Work out the finished part from the listing and answer in its coordinate system (mm). A direction names the side the tool comes from. Round coordinates to 2 decimals unless told otherwise and drop trailing zeros. Write each loop counter-clockwise with the first axis right and the second up, starting at its lowest first coordinate (ties: lowest second). Pieces come first, ordered by that corner, then holes. Notation, with made-up numbers: (11, -15.75) - (49, -15.75) arc R11 ccw to (49, -1.75) - close; hole circle Ø6 at (6, 32). An arc over 180 degrees is marked (long way). Write item = value, one per line. Start each with the question number.
from build123d import *

# Parameters (mm, degrees)
SKETCH_1_R                   = 21.5
EXTRUDE_1_DEPTH              = 12
EXTRUDE_START                = -13.5
EXTRUDE_2_DEPTH              = 13.5
FILLET_1_R                   = 10
SKETCH_4_R                   = 20
CUT_EXTRUDE_1_DEPTH          = 6
SKETCH_5_R                   = 10
CUT_EXTRUDE_2_DEPTH          = 6
SKETCH_6_R                   = 2
EXTRUDE_3_DEPTH              = 3.5
HOLE_WIZARD_M2_1_D           = 1.6
HOLE_WIZARD_M2_1_CSINK_D     = 1.65
HOLE_WIZARD_M2_1_CSINK_ANGLE = 90
CUT_EXTRUDE_3_DEPTH          = 73.320467366
CUT_EXTRUDE_3_DEPTH_BACK     = 23.5
FILLET_2_R                   = 2
FILLET_3_R                   = 2
CHAMFER_1_SIZE               = 1
SKETCH_9_R                   = 1.65
CUT_EXTRUDE_4_DEPTH          = 23.5
CHAMFER_2_SIZE               = 1


with BuildPart() as part:
    # 草图1 → 凸台-拉伸1 (new body)
    with BuildSketch(Plane(origin=(0, 0, 0), x_dir=(1, 0, 0), z_dir=(0, 1, 0))):
        with Locations(Location((0, 0, 0), (0, 0, 270))):
            Circle(SKETCH_1_R)
    extrude(amount=EXTRUDE_1_DEPTH)

    # 草图3 → 凸台-拉伸2 (add)
    with BuildSketch(Plane(origin=(0, 12, 0), x_dir=(1, 0, 0), z_dir=(0, 1, 0)).offset(EXTRUDE_START)):
        with BuildLine():
            Line((-12.5, 46.5), (12.5, 46.5))
            Line((12.5, 46.5), (12.5, 17.492855685))
            ThreePointArc((12.5, 17.492855685), (0, 21.5), (-12.5, 17.492855685))
            Line((-12.5, 17.492855685), (-12.5, 46.5))
        make_face()
    extrude(amount=EXTRUDE_2_DEPTH)

    # 圆角1
    fillet_1_edges = [part.edges().sort_by_distance(p)[0] for p in [
        (12.5, 6, -17.492855685),
        (-12.5, 6, -17.492855685),
    ]]
    fillet(fillet_1_edges, radius=FILLET_1_R)

    # 草图4 → 切除-拉伸1 (cut)
    with BuildSketch(Plane(origin=(0, 0, 0), x_dir=(-1, 0, 0), z_dir=(0, -1, 0))):
        with Locations(Location((0, 0, 0), (0, 0, 90))):
            Circle(SKETCH_4_R)
    extrude(amount=-CUT_EXTRUDE_1_DEPTH, mode=Mode.SUBTRACT)

    # 草图5 → 切除-拉伸2 (cut)
    with BuildSketch(Plane(origin=(0, 6, 0), x_dir=(-1, 0, 0), z_dir=(0, -1, 0))):
        with Locations(Location((0, 0, 0), (0, 0, 90))):
            Circle(SKETCH_5_R)
    extrude(amount=-CUT_EXTRUDE_2_DEPTH, mode=Mode.SUBTRACT)

    # 草图6 → 凸台-拉伸3 (add)
    with BuildSketch(Plane(origin=(0, 6, 0), x_dir=(-1, 0, 0), z_dir=(0, -1, 0))):
        with Locations(Location((14, 0, 0), (0, 0, 90))):
            Circle(SKETCH_6_R)
        with Locations(Location((-7, -12.124355653, 0), (0, 0, 90))):
            Circle(SKETCH_6_R)
        with Locations(Location((-7, 12.124355653, 0), (0, 0, 90))):
            Circle(SKETCH_6_R)
    extrude(amount=EXTRUDE_3_DEPTH)

    # M2 螺纹孔的螺纹孔钻头1 (through all)
    with Locations(Plane(origin=(7, 2.5, 12.124355653), x_dir=(0, 0, -1), z_dir=(0, -1, 0))):
        with Locations((0, 0), (24.248711306, 0), (12.124355653, -21)):
            CounterSinkHole(HOLE_WIZARD_M2_1_D / 2, HOLE_WIZARD_M2_1_CSINK_D / 2, counter_sink_angle=HOLE_WIZARD_M2_1_CSINK_ANGLE)

    # 草图8 → 切除-拉伸3 (cut, two sides: drawn at the far end of the back side and taken through both)
    with BuildSketch(Plane(origin=(0, 0, -46.5), x_dir=(-1, 0, 0), z_dir=(0, 0, -1)).offset(-CUT_EXTRUDE_3_DEPTH_BACK)):
        Polygon((-10.8, 92.015426872), (-10.8, 12), (-10.8, 2.2), (10.8, 2.2), (10.8, 12), (10.8, 92.015426872), (10.8, 252.046280615), (-10.8, 252.046280615), align=None)
    extrude(amount=CUT_EXTRUDE_3_DEPTH + CUT_EXTRUDE_3_DEPTH_BACK, mode=Mode.SUBTRACT)

    # 圆角2
    fillet_2_edges = [part.edges().sort_by_distance(p)[0] for p in [
        (10.8, 7.1, -23),
        (-10.8, 7.1, -23),
    ]]
    fillet(fillet_2_edges, radius=FILLET_2_R)

    # 圆角3
    fillet_3_edges = [part.edges().sort_by_distance(p)[0] for p in [
        (12.5, 5.25, -46.5),
        (-12.5, 5.25, -46.5),
    ]]
    fillet(fillet_3_edges, radius=FILLET_3_R)

    # 倒角1
    chamfer_1_edges = [part.edges().sort_by_distance(p)[0] for p in [
        (0, -1.5, -46.5),
        (-12.5, -1.5, -30.996427842),
        (-11.914213562, -1.5, -45.914213562),
        (11.914213562, -1.5, -45.914213562),
        (12.5, -1.5, -30.996427842),
    ]]
    chamfer(chamfer_1_edges, length=CHAMFER_1_SIZE)

    # 草图9 → 切除-拉伸4 (cut)
    with BuildSketch(Plane(origin=(0, 2.2, 0), x_dir=(1, 0, 0), z_dir=(0, 1, 0))):
        with Locations(Location((-8, 41.5, 0), (0, 0, 270))):
            Circle(SKETCH_9_R)
        with Locations(Location((-8, 28.5, 0), (0, 0, 270))):
            Circle(SKETCH_9_R)
        with Locations(Location((8, 28.5, 0), (0, 0, 270))):
            Circle(SKETCH_9_R)
        with Locations(Location((8, 41.5, 0), (0, 0, 270))):
            Circle(SKETCH_9_R)
    extrude(amount=-CUT_EXTRUDE_4_DEPTH, mode=Mode.SUBTRACT)

    # 倒角2
    chamfer_2_edges = [part.edges().sort_by_distance(p)[0] for p in [
        (8, -1.5, -43.15),
        (8, -1.5, -30.15),
        (-8, -1.5, -30.15),
        (-8, -1.5, -43.15),
    ]]
    chamfer(chamfer_2_edges, length=CHAMFER_2_SIZE)


solid = part.part
1. Find section B-B on x = 0. Give the vertices of the cut face in (y, z), plus the area to 3 significant figures.
2. For a pull along Z with two mould halves and no side action, classify faces 4 (the face through (-12.5, 6, -34)), 5 (the face through (7.601, 4.274, -14.032)), 6 (the face through (0, 7, -23)) as released by +Z, released by -Z, zero draft, split by the parting line, or undercut.
3. Consider line 1 (X direction, y = 8.35, z = 0); line 2 (X direction, y = 3.5, z = -36.5); line 3 (X direction, y = 1, z = 0). Determine where each line is inside the solid, lowest interval first.
4. Find section A-A on y = 3.25. Give the vertices of the cut face in (x, z).
5. Find section D-D on y = 10.25. Give the vertices of the cut face in (x, z), plus the area to 3 significant figures.
6. Each of these flat-tipped pins is pushed along its axis until it touches: pin 1 (1.5 mm diameter, centred on y = 4, z = -39.5, fed in from +X); pin 2 (2 mm diameter, centred on x = -4, y = 4, fed in from -Z); pin 3 (8 mm diameter, centred on y = 7, z = -40, fed in from -X); pin 4 (12 mm diameter, centred on x = 14, z = -20, fed in from +Y). Where does it stop, or does it pass through?
7. Find section C-C on z = -41.5. Give the vertices of the cut face in (x, y).
8. Which of the six approach directions +Z, -Z, +X, -X, +Y, -Y give full straight-line access (tool end or side, diameter ignored) to faces 1 (the face through (0, 2.2, -35)), 2 (the face through (6, 2.5, 12)), 3 (the face through (7.2, 7.3, 12.9))?
Answer key:
q1.outline = (-1.5, -45.5) - (-0.5, -46.5) - (2.2, -46.5) - (2.2, -23) - (12, -23) - (12, -10) - (6, -10) - (6, -20) - (0, -20) - (0, -21.5) - (-1.5, -21.5) - close; (0, 20) - (6, 20) - (6, 10) - (12, 10) - (12, 21.5) - (0, 21.5) - close
q1.area = 263 mm²
q2.face_4 = zero draft
q2.face_5 = undercut
q2.face_6 = released by -Z
q3.line_1 = -21.5 to -14.8, -13.2 to -10, 10 to 21.5
q3.line_2 = -12.5 to -10.8, 10.8 to 12.5
q3.line_3 = -21.5 to -20, 20 to 21.5
q4.outline = circle Ø4 at (-14, 0); (-15.36, -15.05) arc R10 cw to (-12.5, -22.05) - (-12.5, -44.5) arc R2 ccw to (-10.8, -46.48) - (-10.8, -25) arc R2 cw to (-8.8, -23) - (8.8, -23) arc R2 cw to (10.8, -25) - (10.8, -46.48) arc R2 ccw to (12.5, -44.5) - (12.5, -22.05) arc R10 cw to (15.36, -15.05) arc R21.5 ccw (long way) to start; circle Ø4 at (7, -12.12); circle Ø4 at (7, 12.12); hole circle Ø40 at (0, 0); hole circle Ø1.6 at (-14, 0); hole circle Ø1.6 at (7, -12.12); hole circle Ø1.6 at (7, 12.12)
q5.outline = (-15.36, -15.05) arc R10 cw to (-12.5, -22.05) - (-12.5, -44.5) arc R2 ccw to (-10.8, -46.48) - (-10.8, -25) arc R2 cw to (-8.8, -23) - (8.8, -23) arc R2 cw to (10.8, -25) - (10.8, -46.48) arc R2 ccw to (12.5, -44.5) - (12.5, -22.05) arc R10 cw to (15.36, -15.05) arc R21.5 ccw (long way) to start; hole circle Ø1.6 at (-14, 0); hole circle Ø20 at (0, 0); hole circle Ø1.6 at (7, -12.12); hole circle Ø1.6 at (7, 12.12)
q5.area = 1,290 mm²
q6.pin_1 = 12.5
q6.pin_2 = -23
q6.pin_3 = -12.5
q6.pin_4 = 12
q7.outline = (-12.5, -0.5) - (-11.5, -1.5) - (-10.65, -1.5) - (-9.65, -0.5) - (-9.65, 2.2) - (-10.8, 2.2) - (-10.8, 12) - (-12.5, 12) - close; (-6.35, -0.5) - (-5.35, -1.5) - (5.35, -1.5) - (6.35, -0.5) - (6.35, 2.2) - (-6.35, 2.2) - close; (9.65, -0.5) - (10.65, -1.5) - (11.5, -1.5) - (12.5, -0.5) - (12.5, 12) - (10.8, 12) - (10.8, 2.2) - (9.65, 2.2) - close
q8.face_1 = -Z, +Y
q8.face_2 = -Y
q8.face_3 = +Y, -Y
